The drawing under review shows one solid part. Ordinate dimensions are in mm from its lowest x, y, z. A direction names the side the tool comes from. Coordinates: 2 decimals unless noted, no trailing zeros. Order: outer loops, then holes, each group sorted by start corner. A loop starts at its lowest first (then second) coordinate and runs counter-clockwise, first axis right, second up.
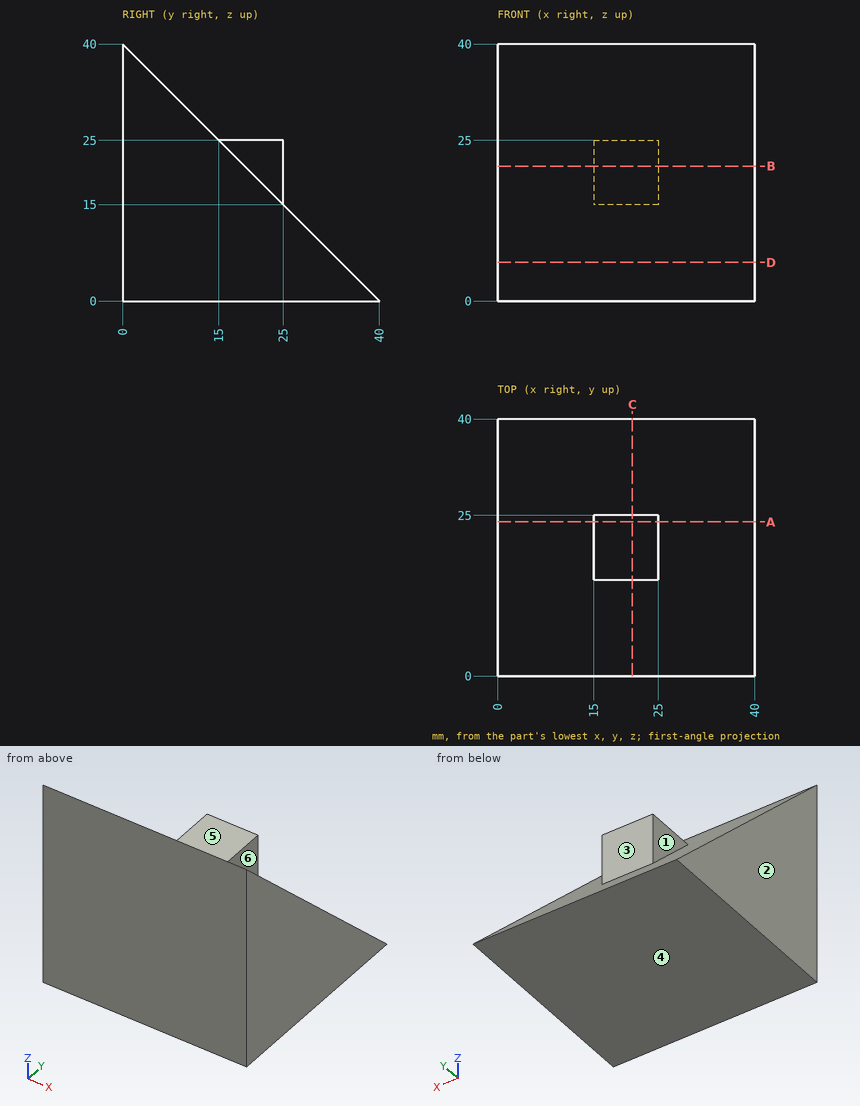
1. Take a section at C-C, the plane x = 21. Give the boundary of the cut face in (y, z), plus the area to 3 significant figures.
Answer below:
outline: (0, 0) - (40, 0) - (25, 15) - (25, 25) - (15, 25) - (0, 40) - close
area: 850 mm2
2. Take a section at B-B, the plane z = 21. Give the boundary of the cut face in (x, y), plus the area to 3 significant figures.
Answer below:
outline: (0, 0) - (40, 0) - (40, 19) - (25, 19) - (25, 25) - (15, 25) - (15, 19) - (0, 19) - close
area: 820 mm2
3. Take a section at D-D, the plane z = 6. Give the boundary of the cut face in (x, y), plus the area to 3 significant figures.
Answer below:
outline: (0, 0) - (40, 0) - (40, 34) - (0, 34) - close
area: 1,360 mm2
4. Clearance check with flat-ended pins moving along their axes: pin 1 Ø2 at (y, z) = (26.5, 17) entering from -X; pin 2 Ø3 at (x, y) = (20, 22) entering from +Z; pin 3 Ø3 at (x, z) = (21, 22) entering from +Y; pin 4 Ø12 at (y, z) = (28.5, 25.5) entering from -X. State where each tip first meets the part, or that it passes through.
Answer below:
pin 1: passes through
pin 2: stops at z = 25
pin 3: stops at y = 25
pin 4: stops at x = 15
5. Machinability: for the marked faces 1, 2 and 3, which of the approach directions +Z, -Z, +X, -X, +Y, -Y give a long, thin tool a straight path to every point of the face, cutting with its end or side? Answer none if there is none.
Answer below:
face 1: +Z, -X, +Y
face 2: +Z, -Z, -X, +Y, -Y
face 3: +Z, +X, -X, +Y
6. To check wall thickness, follow L1, parallel to Y at x = 24, z = 17; L2, parallel to Y at x = 34.5, z = 24.5. State the ranges of each line that lie inside material, in increasing order.
Answer below:
L1: y = 0 to 25
L2: y = 0 to 15.5
7. The part is to be moulded in two halves that separate along Z. For the marked faces 4, 5 and 6, say which applies: +Z half, -Z half, draft (parallel to the pull), parting line (faces both ways), or undercut.
Answer below:
face 4: -Z half
face 5: +Z half
face 6: draft
8. Take a section at A-A, the plane y = 24. Give the boundary of the cut face in (x, z).
Answer below:
outline: (0, 0) - (40, 0) - (40, 16) - (25, 16) - (25, 25) - (15, 25) - (15, 16) - (0, 16) - close
